Can you work these out from the model? Positions are in its coordinate system, mm. A direction names the side the tool comes from. Give positions to 0.01 mm unless a question says otherwise; leave off trailing zeros. Loops run counter-clockwise (first coordinate to the right, second up) from the corner with the lowest first, then second, coordinate; pieces in that order, holes last. Notation, with made-up numbers: (13, -33) - (39, -33) arc R17 ccw to (39, -19) - close; hole circle Ø5 at (-11.75, 86.5). An arc over 180 degrees is marked (long way). Answer in a Markdown table with one row per item.
from build123d import *

# Parameters (mm, degrees)
SKETCH1_R           = 2
BOSS_EXTRUDE1_DEPTH = 4
BOSS_EXTRUDE2_START = -4
BOSS_EXTRUDE2_DEPTH = 4
SKETCH3_R           = 1
CUT_EXTRUDE1_DEPTH  = 6.385164807
SKETCH7_R           = 1
BOSS_EXTRUDE4_DEPTH = 2
SKETCH8_R           = 1
BOSS_EXTRUDE5_DEPTH = 2


with BuildPart() as part:
    # Sketch1 → Boss-Extrude1 (new body)
    with BuildSketch(Plane.XY):
        Circle(SKETCH1_R)
    extrude(amount=BOSS_EXTRUDE1_DEPTH)

    # Sketch2 → Boss-Extrude2 (add)
    with BuildSketch(Plane.XY.offset(4).offset(BOSS_EXTRUDE2_START)):
        with BuildLine():
            Line((3, 2), (0, 2))
            ThreePointArc((0, 2), (1.414213562, 1.414213562), (2, 0))
            ThreePointArc((2, 0), (1.414213562, -1.414213562), (0, -2))
            Line((0, -2), (3, -2))
            Line((3, -2), (3, 2))
        make_face()
    extrude(amount=BOSS_EXTRUDE2_DEPTH)

    # Sketch3 → Cut-Extrude1 (cut, through all)
    with BuildSketch(Plane.XY.offset(4)):
        Circle(SKETCH3_R)
    extrude(amount=-CUT_EXTRUDE1_DEPTH, mode=Mode.SUBTRACT)

    # Sketch7 → Boss-Extrude4 (add, symmetric)
    with BuildSketch(Plane(origin=(0, 0, 0), x_dir=(1, 0, 0), z_dir=(0, 1, 0))):
        with BuildLine():
            Line((3, 0), (3, -4))
            Line((3, -4), (6, -4))
            ThreePointArc((6, -4), (8, -2), (6, 0))
            Line((6, 0), (3, 0))
        make_face()
        with Locations(Location((6, -2, 0), (0, 0, 270))):
            Circle(SKETCH7_R, mode=Mode.SUBTRACT)
    extrude(amount=BOSS_EXTRUDE4_DEPTH, both=True)

    # Sketch8 → Boss-Extrude5 (add)
    with BuildSketch(Plane(origin=(0, 0, 0), x_dir=(1, 0, 0), z_dir=(0, 1, 0))):
        with BuildLine():
            Line((46, -4), (6, -4))
            ThreePointArc((6, -4), (4, -2), (6, 0))
            Line((6, 0), (46, 0))
            ThreePointArc((46, 0), (48, -2), (46, -4))
        make_face()
        with Locations(Location((46, -2, 0), (0, 0, 270))):
            Circle(SKETCH8_R, mode=Mode.SUBTRACT)
        with Locations(Location((6, -2, 0), (0, 0, 270))):
            Circle(SKETCH8_R, mode=Mode.SUBTRACT)
    extrude(amount=BOSS_EXTRUDE5_DEPTH)


solid = part.part
Q1. If we mould it in two halves opening along X, with no side actions, what happens to faces 1 (the face through (48, 1, 2)), 2 (the face through (0, -1, 2)), 3 (the face through (27, 0, 2))? For each: released by +X, released by -X, zero draft, split by the parting line, or undercut.
Checked values:
| item | result |
|---|---|
| face 1 | released by +X |
| face 2 | undercut |
| face 3 | zero draft |
Q2. Imagine slicing it at B-B, the plane x = 40. Write out the boundary of the cut face in (y, z).
Checked values:
| item | result |
|---|---|
| outline | (0, 0) - (2, 0) - (2, 4) - (0, 4) - close |
Q3. If I drill on line 1 (X direction, y = 1.8, z = 2.55); line 2 (X direction, y = 0.6, z = 2); line 3 (X direction, y = 1.5, z = 2), over which ranges is the centre line in solid material (lowest first)? Write a range as [from, to].
Checked values:
| item | result |
|---|---|
| line 1 | x = [-0.87, 5.16], [6.84, 45.16], [46.84, 47.92] |
| line 2 | x = [-1.91, -0.8], [0.8, 5], [7, 45], [47, 48] |
| line 3 | x = [-1.32, 5], [7, 45], [47, 48] |
Q4. On a 3-axis mill with a long thin cutter (end or side, diameter ignored), from which of +Z, -Z, +X, -X, +Y, -Y can I reach the whole of each face in a straight line? I mean faces 4 (the face through (8, -1, 2)), 5 (the face through (22, 1, 0)). Say none if no direction works.
Checked values:
| item | result |
|---|---|
| face 4 | +X, -Y |
| face 5 | -Z, +X, -X, +Y, -Y |
Q5. Imagine slicing it at A-A, the plane z = 2. Write out the boundary of the cut face in (x, y), and give its area (3 significant figures).
Checked values:
| item | result |
|---|---|
| outline | (0, -2) - (5, -2) - (5, 2) - (0, 2) arc R2 ccw to start; (7, -2) - (8, -2) - (8, 0) - (45, 0) - (45, 2) - (7, 2) - close; (47, 0) - (48, 0) - (48, 2) - (47, 2) - close; hole circle Ø2 at (0, 0) |
| area | 103 mm² |
Q6. For pin 1 (2 mm diameter, centred on y = 0.5, z = 2.5, fed in from +X); pin 2 (2 mm diameter, centred on x = 23.5, z = 2, fed in from -Y), each with a flat end and sliding along its axis, tell me the tip position at first contact or that it passes through.
Checked values:
| item | result |
|---|---|
| pin 1 | stops at x = 48 |
| pin 2 | stops at y = 0 |
Q7. Imagine slicing it at C-C, the plane y = 1.5. Write out the boundary of the cut face in (x, z), and give its area (3 significant figures).
Checked values:
| item | result |
|---|---|
| outline | (-1.32, 0) - (46, 0) arc R2 ccw to (46, 4) - (-1.32, 4) - close; hole circle Ø2 at (6, 2); hole circle Ø2 at (46, 2) |
| area | 189 mm² |
